The listing builds one solid part. Answer for the finished solid, in the listing's coordinates (mm). A direction names the side the tool comes from. Round coordinates to 2 decimals unless told otherwise and drop trailing zeros. Loops run counter-clockwise (first coordinate to the right, second up) from the corner with the lowest first, then second, coordinate; pieces in that order, holes last. Notation, with made-up numbers: (54.25, -39.5) -> (101.25, -39.5) arc R19 cw to (101.25, -26.5) -> close; hole circle Ø3 at (-6.5, -29). An arc over 180 degrees is marked (long way). Use a Markdown table: item, result. Add a question column.
Q1. For a pull along X with two mould halves and no side action, classify faces 4 (the flat face through (-13, 201, 10)), 5 (the cylindrical face through (0, 128, 18)), 6 (the cylindrical face through (-15.62, 206.92, -3.47)) as released by +X, released by -X, zero draft, split by the parting line, or undercut.
Q2. Section C-C on y = 170.5 is taken. Give the vertices of the cut face in (x, z).
Q3. Which of the six approach directions +Z, -Z, +X, -X, +Y, -Y give full straight-line access (tool end or side, diameter ignored) to faces 1 (the flat face through (-6, 144, 18)), 2 (the flat face through (0, 35, 13.5)), 3 (the flat face through (20.5, 162, -5.7))?
Q4. Section B-B on z = 0 is taken. Give the vertices of the cut face in (x, y), then the cut area to 3 significant figures.
Q5. Consider line 1 (X direction, y = 156.5, z = 0); line 2 (X direction, y = 109, z = 1); line 3 (Y direction, x = -11.5, z = -8). Determine where each line is inside the solid, lowest interval first.
Q6. Given pin 1 Ø2 at (y, z) = (142.5, 13.5) entering from -X; pin 2 Ø2 at (x, y) = (-15.5, 182) entering from -Z; pin 3 Ø2 at (y, z) = (103.5, 4) entering from -X; pin 4 Ø25 at (x, z) = (0.5, 3) entering from -Y, each flat-ended and moving along its own axis, determine where each tip first touches the part or whether it passes through.
Q7. Section D-D on y = 77.5 is taken. Give the vertices of the cut face in (x, z).
from build123d import *

# Parameters (mm, degrees)
F2_SIZE  = 1
F3_SIZE  = 2
F6_DEPTH = 11.501
F9_DEPTH = 9.001


with BuildPart() as f1:
    # F0 (on Right) → F1 (revolve)
    with BuildSketch(Plane.YZ):
        Polygon((0, 18.5), (0, 0), (215, 0), (215, 16), (201, 16), (201, 19), (166, 19), (166, 25), (162, 25), (162, 21), (125, 21), (125, 20), (75, 20), (75, 18.5), align=None)
    revolve(axis=Axis((0, 105.03928, 0), (0, 1, 0)))

    # F2
    f2_edges = [f1.edges().sort_by_distance(p)[0] for p in [
        (0, 0, -18.5),
    ]]
    chamfer(f2_edges, length=F2_SIZE)

    # F3
    f3_edges = [f1.edges().sort_by_distance(p)[0] for p in [
        (0, 215, -16),
    ]]
    chamfer(f3_edges, length=F3_SIZE)

    # F5 (on offset) → F6 (cut, through all)
    with BuildSketch(Plane.XY.offset(13.5)):
        with BuildLine():
            Line((5, -5), (5, 65))
            ThreePointArc((5, 65), (0, 70), (-5, 65))
            Line((-5, 65), (-5, -5))
            Line((-5, -5), (0, -5))
            Line((0, -5), (5, -5))
        make_face()
    extrude(amount=F6_DEPTH, mode=Mode.SUBTRACT)

    # F8 (on offset) → F9 (cut, through all)
    with BuildSketch(Plane.XY.offset(16)):
        with BuildLine():
            Line((6, 134), (6, 154))
            ThreePointArc((6, 154), (0, 160), (-6, 154))
            Line((-6, 154), (-6, 134))
            ThreePointArc((-6, 134), (0, 128), (6, 134))
        make_face()
    extrude(amount=F9_DEPTH, mode=Mode.SUBTRACT)


solid = f1.part
Checked values:
| question | item | result |
|---|---|---|
| 1 | face 4 | zero draft |
| 1 | face 5 | undercut |
| 1 | face 6 | split by the parting line |
| 2 | outline | circle Ø38 at (0, 0) |
| 3 | face 1 | +Z |
| 3 | face 2 | +Z, -Y |
| 3 | face 3 | -Y |
| 4 | outline | (-25, 162) -> (-21, 162) -> (-21, 125) -> (-20, 125) -> (-20, 75) -> (-18.5, 75) -> (-18.5, 1) -> (-17.5, 0) -> (17.5, 0) -> (18.5, 1) -> (18.5, 75) -> (20, 75) -> (20, 125) -> (21, 125) -> (21, 162) -> (25, 162) -> (25, 166) -> (19, 166) -> (19, 201) -> (16, 201) -> (16, 213) -> (14, 215) -> (-14, 215) -> (-16, 213) -> (-16, 201) -> (-19, 201) -> (-19, 166) -> (-25, 166) -> close |
| 4 | area | 8,300 mm2 |
| 5 | line 1 | x = -21 to 21 |
| 5 | line 2 | x = -19.97 to 19.97 |
| 5 | line 3 | y = 0 to 214.99 |
| 6 | pin 1 | stops at x = -16.87 |
| 6 | pin 2 | stops at z = -12.28 |
| 6 | pin 3 | stops at x = -19.77 |
| 6 | pin 4 | stops at y = 0 |
| 7 | outline | circle Ø40 at (0, 0) |
